```python
from build123d import *

# Parameters (mm, degrees)
SKETCH1_R           = 5.1
BOSS_EXTRUDE1_DEPTH = 1
BOSS_EXTRUDE2_START = 0.5
SKETCH2_R           = 0.5
BOSS_EXTRUDE2_DEPTH = 1


with BuildPart() as part:
    # Sketch1 → Boss-Extrude1 (new body)
    with BuildSketch(Plane(origin=(0, 0, 0), x_dir=(0, 0, -1), z_dir=(1, 0, 0))):
        Circle(SKETCH1_R)
    extrude(amount=BOSS_EXTRUDE1_DEPTH)

    # Sketch2 → Boss-Extrude2 (add)
    with BuildSketch(Plane(origin=(0, 0, 0), x_dir=(1, 0, 0), z_dir=(0, 1, 0)).offset(BOSS_EXTRUDE2_START)):
        with BuildLine():
            Line((1, 1), (2, 1))
            ThreePointArc((2, 1), (3, 0), (2, -1))
            Line((2, -1), (1, -1))
            Line((1, -1), (1, 1))
        make_face()
        with Locations((2, 0)):
            Circle(SKETCH2_R, mode=Mode.SUBTRACT)
    boss_extrude2 = extrude(amount=BOSS_EXTRUDE2_DEPTH)

    # Mirror1: Boss-Extrude2 across plane
    add(boss_extrude2.mirror(Plane.ZX))


solid = part.part
```
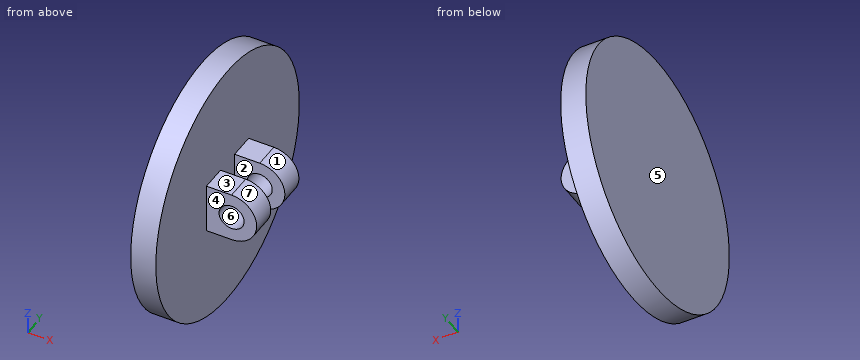
Design review of the part built by this model. Coordinates are the model's own, in mm. Face numbers are marked on the shaded views. A direction names the side the tool comes from. Coordinates: 2 decimals unless noted, no trailing zeros. Order: outer loops, then holes, each group sorted by start corner. A loop starts at its lowest first (then second) coordinate and runs counter-clockwise, first axis right, second up. Notation, with made-up numbers: (56.5, 78) - (102.5, 78) arc R8 ccw to (102.5, 88) - close; hole circle Ø10 at (75, 15). An arc over 180 degrees is marked (long way). Answer in a Markdown table with one row per item.
(1) Wall thickness on line 1 along X through (y, z) = (-0.75, 0); line 2 along Z through (x, y) = (2, -1.25); line 3 along Y through (x, z) = (2.8, -0.25): over which ranges is each line inside the solid? List them lowest first. Write a range as from..to.
Checked values:
| item | result |
|---|---|
| line 1 | 0..1.5, 2.5..3 |
| line 2 | -1..-0.5, 0.5..1 |
| line 3 | -1.5..-0.5, 0.5..1.5 |
(2) For the marked faces 1, 2 and 3, list the 3-axis set-ups (+Z, -Z, +X, -X, +Y, -Y) from which the entire face can be reached by the end or side of a thin tool; tool diameter is ignored.
Checked values:
| item | result |
|---|---|
| face 1 | +X, +Y, -Y |
| face 2 | +Z, -Z, +X |
| face 3 | +Z, +X, +Y, -Y |
(3) Consider section C-C on x = 0.85. State the section outline as (y, z) points, plus the area to 3 significant figures.
Checked values:
| item | result |
|---|---|
| outline | circle Ø10.2 at (0, 0) |
| area | 81.7 mm^2 |
(4) Consider section A-A on z = 0. State the section outline as (x, y) points, plus the area to 3 significant figures.
Checked values:
| item | result |
|---|---|
| outline | (0, -5.1) - (1, -5.1) - (1, -1.5) - (1.5, -1.5) - (1.5, -0.5) - (1, -0.5) - (1, 0.5) - (1.5, 0.5) - (1.5, 1.5) - (1, 1.5) - (1, 5.1) - (0, 5.1) - close; (2.5, -1.5) - (3, -1.5) - (3, -0.5) - (2.5, -0.5) - close; (2.5, 0.5) - (3, 0.5) - (3, 1.5) - (2.5, 1.5) - close |
| area | 12.2 mm^2 |
(5) Clearance check with flat-ended pins moving along their axes: pin 1 (1.6 mm diameter, centred on x = 2, z = 0, fed in from +Y); pin 2 (0.6 mm diameter, centred on x = 2, z = -0.5, fed in from -Y); pin 3 (1 mm diameter, centred on x = 2.5, y = -3.5, fed in from +Z); pin 4 (0.5 mm diameter, centred on x = 1.5, y = -1, fed in from -Z). State where each tip first meets the part, or that it passes through.
Checked values:
| item | result |
|---|---|
| pin 1 | y = 1.5 |
| pin 2 | y = -1.5 |
| pin 3 | through |
| pin 4 | z = -1 |
(6) Consider section B-B on x = 1.8. State the section outline as (y, z) points.
Checked values:
| item | result |
|---|---|
| outline | (-1.5, -1) - (-0.5, -1) - (-0.5, -0.46) - (-1.5, -0.46) - close; (-1.5, 0.46) - (-0.5, 0.46) - (-0.5, 1) - (-1.5, 1) - close; (0.5, -1) - (1.5, -1) - (1.5, -0.46) - (0.5, -0.46) - close; (0.5, 0.46) - (1.5, 0.46) - (1.5, 1) - (0.5, 1) - close |
(7) The part is to be moulded in two halves that separate along X. For the marked faces 4, 5, 6 and 7, say which applies: released by +X, released by -X, zero draft, split by the parting line, or undercut.
Checked values:
| item | result |
|---|---|
| face 4 | zero draft |
| face 5 | released by -X |
| face 6 | undercut |
| face 7 | released by +X |
(8) Consider section D-D on y = 0. State the section outline as (x, z) points.
Checked values:
| item | result |
|---|---|
| outline | (0, -5.1) - (1, -5.1) - (1, 5.1) - (0, 5.1) - close |
